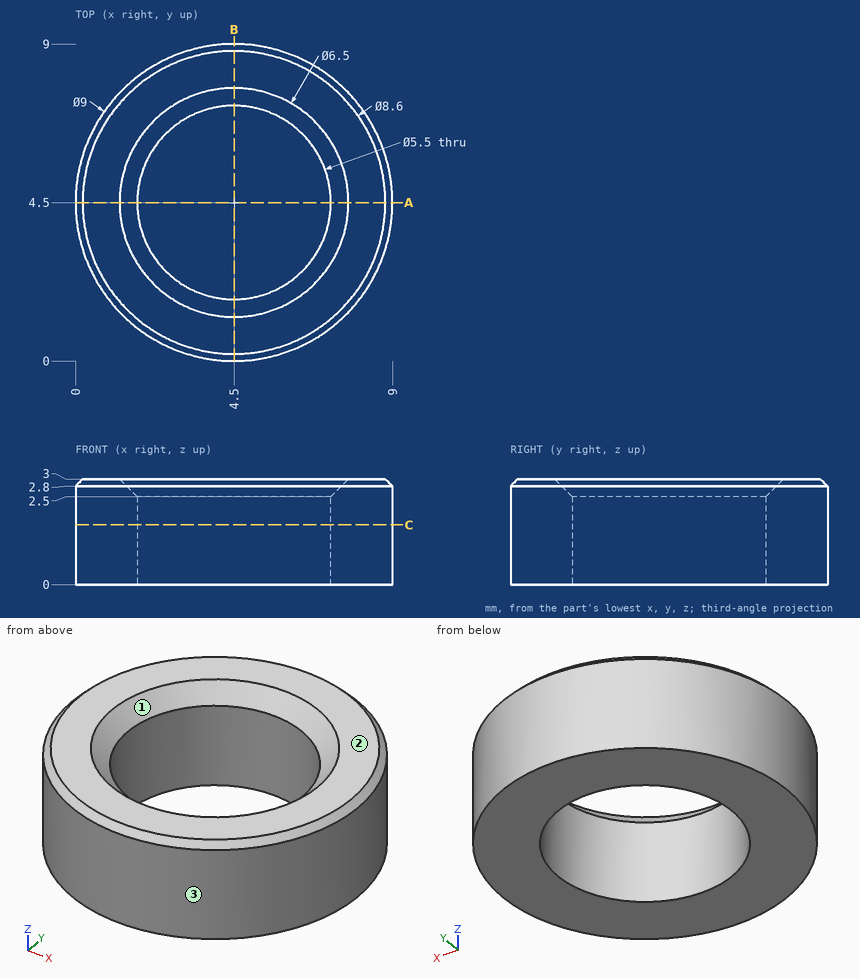
Check sheet for the drawn part. Datum: minimum x, y, z corner. Units: mm. Round coordinates to 2 decimals unless told otherwise and drop trailing zeros. Loops run counter-clockwise (first coordinate to the right, second up) from the corner with the lowest first, then second, coordinate; pieces in that order, holes last. Notation, with made-up numbers: M 35,55 L 40,55 A21 cw 40,94 Z; hole C 58,39 d6. An arc over 180 degrees is marked long. One line per question, with ' | ' between items. Start each with the question number.
Item 1: Section check C-C (z = 1.7). Record the boundary of the cut face in (x, y).
Item 2: Section check A-A (y = 4.5). Record the boundary of the cut face in (x, z), and give its area (3 significant figures).
Item 3: Release check for a two-part mould opening along Y. For the marked faces 1, 2 and 3 record: released by +Y, released by -Y, zero draft, split by the parting line, or undercut.
Item 4: Scan lines: probe 1 along Y at (x, z) = (4.5, 1.9); probe 2 along X at (y, z) = (7, 0.2); probe 3 along Y at (x, z) = (6, 1.05). Record each from-to range of solid material in increasing order.
Worked out:
1) outline: C 4.5,4.5 d9; hole C 4.5,4.5 d5.5
2) outline: M 0,0 L 1.75,0 L 1.75,2.5 L 1.25,3 L 0.2,3 L 0,2.8 Z; M 7.25,0 L 9,0 L 9,2.8 L 8.8,3 L 7.75,3 L 7.25,2.5 Z | area: 10.2 mm^2
3) face 1: undercut | face 2: zero draft | face 3: split by the parting line
4) probe 1: 0 to 1.75, 7.25 to 9 | probe 2: 0.76 to 3.35, 5.65 to 8.24 | probe 3: 0.26 to 2.2, 6.8 to 8.74
